Part model, mm, in its own coordinate system. A direction names the side the tool comes from. Coordinates: 2 decimals unless noted, no trailing zeros. Loops run counter-clockwise (first coordinate to the right, second up) from the corner with the lowest first, then second, coordinate; pieces in that order, holes last. Notation, with made-up numbers: M 8,-13 L 58,-13 A22 cw 58,7 Z; hole C -28,-6 d6. An arc over 180 degrees is marked long. Answer as CSV lines item,"result". Start each with the question number.
from build123d import *

# Parameters (mm, degrees)
F0_W     = 85
F0_H     = 75
F1_DEPTH = 5
F3_DEPTH = 15


with BuildPart() as f1:
    # F0 (on Top) → F1 (new body)
    with BuildSketch(Plane.XY):
        with Locations((-27.537888, 6.086919)):
            Rectangle(F0_W, F0_H)
    extrude(amount=F1_DEPTH)

    # F2 (on face) → F3 (join)
    with BuildSketch(Plane(origin=(0, 0, 0), x_dir=(1, 0, 0), z_dir=(0, 0, -1))):
        with BuildLine():
            ThreePointArc((-47.554573, -29.086919), (-47.542061, -28.837059), (-47.537888, -28.586919))
            ThreePointArc((-47.537888, -28.586919), (-47.542061, -28.33678), (-47.554573, -28.086919))
            ThreePointArc((-47.554573, -28.086919), (-49.734587, -23.283619), (-54.537888, -21.103605))
            ThreePointArc((-54.537888, -21.103605), (-55.037888, -21.086919), (-55.537888, -21.103605))
            ThreePointArc((-55.537888, -21.103605), (-60.342111, -23.284541), (-62.521376, -28.089523))
            ThreePointArc((-62.521376, -28.089523), (-62.537888, -28.589529), (-62.521028, -29.089523))
            ThreePointArc((-62.521028, -29.089523), (-60.340266, -33.891143), (-55.537888, -36.070234))
            ThreePointArc((-55.537888, -36.070234), (-55.037888, -36.086919), (-54.537888, -36.070234))
            ThreePointArc((-54.537888, -36.070234), (-49.734587, -33.89022), (-47.554573, -29.086919))
        make_face()
        with BuildLine():
            ThreePointArc((-62.521028, -29.089523), (-62.537888, -28.589529), (-62.521376, -28.089523))
            Line((-62.521376, -28.089523), (-63.537888, -28.089523))
            Line((-63.537888, -28.089523), (-63.537888, -29.089523))
            Line((-63.537888, -29.089523), (-62.521028, -29.089523))
        make_face()
        with BuildLine():
            ThreePointArc((-47.554573, -28.086919), (-47.542061, -28.33678), (-47.537888, -28.586919))
            ThreePointArc((-47.537888, -28.586919), (-47.542061, -28.837059), (-47.554573, -29.086919))
            Line((-47.554573, -29.086919), (-46.537888, -29.086919))
            Line((-46.537888, -29.086919), (-46.537888, -28.086919))
            Line((-46.537888, -28.086919), (-47.554573, -28.086919))
        make_face()
        with BuildLine():
            ThreePointArc((-55.537888, -21.103605), (-55.037888, -21.086919), (-54.537888, -21.103605))
            Line((-54.537888, -21.103605), (-54.537888, -20.086919))
            Line((-54.537888, -20.086919), (-55.537888, -20.086919))
            Line((-55.537888, -20.086919), (-55.537888, -21.103605))
        make_face()
        with BuildLine():
            Line((-54.537888, -37.086919), (-54.537888, -36.070234))
            ThreePointArc((-54.537888, -36.070234), (-55.037888, -36.086919), (-55.537888, -36.070234))
            Line((-55.537888, -36.070234), (-55.537888, -37.086919))
            Line((-55.537888, -37.086919), (-54.537888, -37.086919))
        make_face()
    extrude(amount=F3_DEPTH)


solid = f1.part
Q1. Wall check: L1, parallel to Z at x = 3.5, y = 37; L2, parallel to X at y = 24, z = -7.25; L3, parallel to Y at x = -63.5, z = -7.25. Give the ranges that are in metal, low to high.
Q2. Slice it at B-B, the plane x = -26. Write the cut outline in (y, z).
Q3. Slice it at C-C, the plane y = 38.5. Write the cut outline in (x, z).
Q4. Tool access for faces 1 (the face through (-60.288, 23.231, -7.395)), 2 (the face through (-49.788, 33.943, -7.395)), 3 (the face through (-60.39, 33.84, -7.4)), 4 (the face through (-49.68, 23.34, -7.4)): list every direction of +Z, -Z, +X, -X, +Y, -Y with a clear straight run to the whole face (end or side of a thin tool).
Q5. Slice it at A-A, the plane z = -6. Write the cut outline in (x, y), and give its area (3 significant figures).
Q6. Flat gauge pins, fed straight in: P1, Ø10, axis at x = 5.5, y = 5, coming from the -Z side; P2, Ø0.5, axis at x = -47, z = -10, coming from the +Y side; P3, Ø0.5, axis at x = -55, z = -9, coming from the +Y side; P4, Ø12, axis at x = -5, z = -10.5, coming from the +Y side. Where does each tip first touch, or does it go through?
Solved:
1,L1,"z = 0 to 5"
1,L2,"x = -60.97 to -49.1"
1,L3,"y = 28.09 to 29.09"
2,outline,"M -31.41,0 L 43.59,0 L 43.59,5 L -31.41,5 Z"
3,outline,"M -70.04,0 L 14.96,0 L 14.96,5 L -70.04,5 Z"
4,face 1,"-Z, -X, -Y"
4,face 2,"-Z, +X, +Y"
4,face 3,"-Z, -X, +Y"
4,face 4,"-Z, +X, -Y"
5,outline,"M -63.54,28.09 L -62.52,28.09 A7.5 ccw -55.54,21.1 L -55.54,20.09 L -54.54,20.09 L -54.54,21.1 A7.5 ccw -47.55,28.09 L -46.54,28.09 L -46.54,29.09 L -47.55,29.09 A7.5 ccw -54.54,36.07 L -54.54,37.09 L -55.54,37.09 L -55.54,36.07 A7.5 ccw -62.52,29.09 L -63.54,29.09 Z"
5,area,"181 mm2"
6,P1,"stops at z = 0"
6,P2,"stops at y = 29.09"
6,P3,"stops at y = 37.09"
6,P4,"passes through"
